For this review, take the finished solid that the model builds, in its own axes (mm). Face numbers are marked on the shaded views. A direction names the side the tool comes from. Coordinates: 2 decimals unless noted, no trailing zeros. Loops run counter-clockwise (first coordinate to the right, second up) from the corner with the lowest first, then second, coordinate; pieces in that order, holes last. Notation, with made-up numbers: (89, 73.5) - (114, 73.5) arc R11 cw to (114, 82.5) - close; hole circle Ø7 at (12.25, 28). An arc over 180 degrees is marked (long way). Use one line per item in the form item = value. Start each with the question number.
1. Add section A-A on z = 0. Count the separate pieces of the cut face and the enclosed holes in it, and give its area (3 significant figures).
2. Add section D-D on x = -48. Give the boundary of the cut face in (y, z), and give its area (3 significant figures).
3. Machinability: for the marked faces 4, 5, 6, 7 and 8, which of the approach directions +Z, -Z, +X, -X, +Y, -Y give a long, thin tool a straight path to every point of the face, cutting with its end or side? Answer none if there is none.
4. Add section C-C on y = 55. Give the boundary of the cut face in (x, z).
5. To check wall thickness, follow probe 1 along Z at (x, y) = (1, -30); probe 2 along X at (y, z) = (23, -1.5); probe 3 along Z at (x, y) = (-9, 62.5). State the ranges of each line that lie inside material, in increasing order.
6. Draft analysis for pull direction Y (two halves, no side actions). For the marked faces 1, 2 and 3, state which applies: +Y half, -Y half, draft (parallel to the pull), parting line (faces both ways), or undercut.
7. For pin 1 Ø3 at (y, z) = (55.5, -3.5) entering from +X; pin 2 Ø5 at (y, z) = (25.5, -2) entering from +X; pin 3 Ø3 at (y, z) = (42.5, 0.5) entering from -X; pin 4 Ø3 at (x, y) = (35, 55) entering from +Z, all flat-tipped, find the tip position at first contact; note any pin that passes through.
8. Add section B-B on y = -30. Give the boundary of the cut face in (x, z), and give its area (3 significant figures).
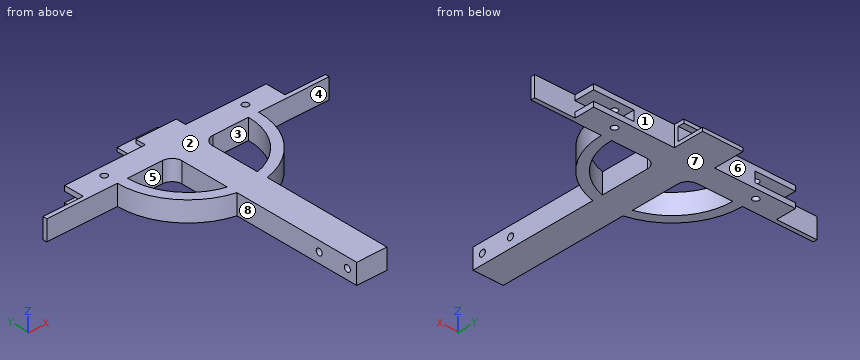
```python
from build123d import *

# Parameters (mm, degrees)
F0_W      = 15
F0_H      = 100
F1_DEPTH  = 5
F2_W      = 100
F2_H      = 10
F3_DEPTH  = 10
F4_W      = 10
F4_H      = 5
F5_DEPTH  = 20
F6_W      = 10
F6_H      = 5
F7_DEPTH  = 20
F8_R      = 1.6
F9_DEPTH  = 10
F10_W     = 77.5
F10_H     = 10
F10_W_2   = 140
F11_DEPTH = 2
F12_R     = 5
F13_R     = 1.6
F14_DEPTH = 15
F15_W     = 20
F15_H     = 10
F16_DEPTH = 5
F17_W     = 20
F17_H     = 6.5
F18_DEPTH = 3
F19_DEPTH = 10
F21_DEPTH = 10


# Not quite as in the source:
# - a pattern or mirror of a feature is missing from the dataset's text; its kind, count and spacing are read off the source's solid


with BuildPart() as f1:
    # F0 (on Top) → F1 (new body, symmetric)
    with BuildSketch(Plane.XY):
        Rectangle(F0_W, F0_H)
    extrude(amount=F1_DEPTH, both=True)

    # F2 (on face) → F3 (join)
    with BuildSketch(Plane(origin=(0, 50, 0), x_dir=(-1, 0, 0), z_dir=(0, 1, 0))):
        Rectangle(F2_W, F2_H)
    extrude(amount=F3_DEPTH)

    # F4 (on face) → F5 (cut)
    with BuildSketch(Plane(origin=(-50, 0, 0), x_dir=(0, -1, 0), z_dir=(-1, 0, 0))):
        with Locations((-55, 0)):
            Rectangle(F4_W, F4_H)
    extrude(amount=-F5_DEPTH, mode=Mode.SUBTRACT)

    # F6 (on face) → F7 (cut)
    with BuildSketch(Plane.YZ.offset(50)):
        with Locations((55, 0)):
            Rectangle(F6_W, F6_H)
    extrude(amount=-F7_DEPTH, mode=Mode.SUBTRACT)

    # F8 (on face) → F9 (cut, through all)
    with BuildSketch(Plane.XY.offset(5)):
        with Locations((-35, 55)):
            Circle(F8_R)
        with Locations((35, 55)):
            Circle(F8_R)
    extrude(amount=-F9_DEPTH, mode=Mode.SUBTRACT)

    # F10 (on face) → F11 (join)
    with BuildSketch(Plane.XZ.offset(-50)):
        with Locations((31.25, 0)):
            Rectangle(F10_W, F10_H)
        Rectangle(F10_W_2, F10_H)
    extrude(amount=F11_DEPTH)

    # F12
    f12_edges = [f1.edges().sort_by_distance(p)[0] for p in [
        (-7.5, 48, 0),
        (7.5, 48, 0),
    ]]
    fillet(f12_edges, radius=F12_R)

    # F13 (on face) → F14 (cut, through all)
    with BuildSketch(Plane(origin=(-7.5, 0, 0), x_dir=(0, -1, 0), z_dir=(-1, 0, 0))):
        with Locations((30, 0)):
            Circle(F13_R)
        with Locations((45, 0)):
            Circle(F13_R)
    extrude(amount=-F14_DEPTH, mode=Mode.SUBTRACT)

    # F15 (on face) → F16 (join)
    with BuildSketch(Plane(origin=(0, 60, 0), x_dir=(-1, 0, 0), z_dir=(0, 1, 0))):
        Rectangle(F15_W, F15_H)
    extrude(amount=F16_DEPTH)

    # F17 (on face) → F18 (cut)
    with BuildSketch(Plane(origin=(0, 65, 0), x_dir=(-1, 0, 0), z_dir=(0, 1, 0))):
        Rectangle(F17_W, F17_H)
    extrude(amount=-F18_DEPTH, mode=Mode.SUBTRACT)

    # F19 (add): a face of the model
    f19_faces = [f1.faces().sort_by_distance(p)[0] for p in [
        (0, 65, -4.125),
    ]]
    extrude(f19_faces, amount=F19_DEPTH)

    # F20 (on face) → F21 (join, through all)
    with BuildSketch(Plane.XY.offset(5)):
        with BuildLine():
            Line((35, 48), (30, 48))
            ThreePointArc((30, 48), (23.7170824513, 29.6288269291), (7.5, 18.9526249034))
            Line((7.5, 18.9526249034), (7.5, 13.8130141721))
            ThreePointArc((7.5, 13.8130141721), (27.2717802866, 26.0625890315), (35, 48))
        make_face()
    f21 = extrude(amount=-F21_DEPTH)

    # F21_copies: F21 across plane
    add(f21.mirror(Plane(origin=(0, 0, 0), x_dir=(0, 0, -1), z_dir=(-1, 0, 0))))


solid = f1.part
```
Conclusion:
q1.separate_pieces = 3
q1.enclosed_holes = 2
q1.area = 2,740 mm^2
q2.outline = (48, -5) - (60, -5) - (60, -2.5) - (50, -2.5) - (50, 2.5) - (60, 2.5) - (60, 5) - (48, 5) - close
q2.area = 70.0 mm^2
q3.face_4 = +Z, -Z, +X, -Y
q3.face_5 = +Z, -Z
q3.face_6 = +Z, -Z, -X, +Y
q3.face_7 = -Z, +X, -X, +Y, -Y
q3.face_8 = +Z, -Z, -X, -Y
q4.outline = (-50, -5) - (-36.6, -5) - (-36.6, -2.5) - (-50, -2.5) - close; (-50, 2.5) - (-36.6, 2.5) - (-36.6, 5) - (-50, 5) - close; (-33.4, -5) - (33.4, -5) - (33.4, -2.5) - (30, -2.5) - (30, 2.5) - (33.4, 2.5) - (33.4, 5) - (-33.4, 5) - (-33.4, 2.5) - (-30, 2.5) - (-30, -2.5) - (-33.4, -2.5) - close; (36.6, -5) - (50, -5) - (50, -2.5) - (36.6, -2.5) - close; (36.6, 2.5) - (50, 2.5) - (50, 5) - (36.6, 5) - close
q5.probe_1 = -5 to -1.6, 1.6 to 5
q5.probe_2 = -24.49 to -16.58, -7.5 to 7.5, 16.58 to 24.49
q5.probe_3 = -5 to -3.25, 3.25 to 5
q6.face_1 = +Y half
q6.face_2 = draft
q6.face_3 = undercut
q7.pin_1 = 50
q7.pin_2 = 28.72
q7.pin_3 = -34.77
q7.pin_4 = through
q8.outline = (-7.5, -5) - (7.5, -5) - (7.5, -1.6) - (-7.5, -1.6) - close; (-7.5, 1.6) - (7.5, 1.6) - (7.5, 5) - (-7.5, 5) - close
q8.area = 102 mm^2
